The model under review builds one solid part; all positions refer to its coordinate system, in mm. A direction names the side the tool comes from. Coordinates: 2 decimals unless noted, no trailing zeros. Loops run counter-clockwise (first coordinate to the right, second up) from the corner with the lowest first, then second, coordinate; pieces in that order, holes last. Notation, with made-up numbers: (17, -9) - (54, -9) arc R18 cw to (54, 9) - close; hole circle Ø4 at (-24.5, -25). An arc over 180 degrees is marked (long way). Answer in a Markdown table with one row per item. Add a question column.
(1) Mouldability with a two-part tool opening along Y and no side actions: class faces 1 (the flat face through (29.689, 15.675, -12.567)), 2 (the conical face through (-20.821, -93.761, 28.116)), 3 (the flat face through (-8, -77, 28.575)) as +Y half, -Y half, draft (parallel to the pull), parting line (faces both ways), or undercut.
(2) For P1, Ø4, axis at x = -70.5, z = -17.5, coming from the -Y side; P2, Ø6, axis at x = -79, z = 5, coming from the -Y side; P3, Ø15, axis at y = 38, z = -11.5, coming from the +X side, all flat-tipped, find the tip position at first contact; note any pin that passes through.
(3) We need section A-A on z = 18.5. Write out the cut boundary in (x, y) (3 decimals), plus the area to 3 significant figures.
(4) Machinability: for faces 4 (the flat face through (-1.27, 33, -13)), 5 (the cylindrical face through (50.8, -0.4, 12.8)), which of the approach directions +Z, -Z, +X, -X, +Y, -Y give a long, thin tool a straight path to every point of the face, cutting with its end or side? Answer none if there is none.
(5) For line 1 along X through (y, z) = (1, 5.5); line 2 along X through (y, z) = (24, 9); line 3 along X through (y, z) = (-18.5, -4), list the stretches that pass through material, from the lowest coordinate up.
from build123d import *
from OCP.BRepFilletAPI import BRepFilletAPI_MakeChamfer

# Parameters (mm, degrees)
EXTRUDE1_DEPTH          = 28.575
EXTRUDE1_DEPTH_BACK     = 28.575
SKETCH1_R               = 107.95
CHAMFER1_SIZE           = 12.7
CHAMFER1_SIZE2          = 7.332348419
SKETCH2_R               = 60.325
EXTRUDE2_DEPTH          = 6.35
FILLET1_R               = 25.4
SKETCH5_R               = 50.8
EXTRUDE4_DEPTH          = 19.05
SKETCH6_W               = 2.54
SKETCH6_H               = 50.8
EXTRUDE_THIN1_DEPTH     = 19.05
CIRPATTERN2_COUNT       = 6
SKETCH7_R               = 15.875
EXTRUDE5_DEPTH          = 19.05
MIRROR4_COPY_1_SKETCH_W = 2.54
MIRROR4_COPY_1_SKETCH_H = 50.8
MIRROR4_COPY_1_DEPTH    = 19.05
MIRROR4_COPY_2_SKETCH_W = 2.54
MIRROR4_COPY_2_SKETCH_H = 50.8
MIRROR4_COPY_2_DEPTH    = 19.05
MIRROR4_COPY_3_SKETCH_W = 2.54
MIRROR4_COPY_3_SKETCH_H = 50.8
MIRROR4_COPY_3_DEPTH    = 19.05
MIRROR4_COPY_4_SKETCH_W = 2.54
MIRROR4_COPY_4_SKETCH_H = 50.8
MIRROR4_COPY_4_DEPTH    = 19.05
MIRROR4_COPY_5_SKETCH_W = 2.54
MIRROR4_COPY_5_SKETCH_H = 50.8
MIRROR4_COPY_5_DEPTH    = 19.05
FILLET2_R               = 25.4


with BuildPart() as part:
    # Sketch1 → Extrude1 (new, two sides: drawn at the far end of the back side and taken through both)
    with BuildSketch(Plane.XY.offset(-EXTRUDE1_DEPTH_BACK)):
        Circle(SKETCH1_R)
    extrude(amount=EXTRUDE1_DEPTH + EXTRUDE1_DEPTH_BACK)

    # Chamfer1: one chamfer whose edges measure the first distance from different faces: ONE call of the kernel's chamfer builder (chamfer() names one face for all edges)
    chamfer1_edges_1 = [part.edges().sort_by_distance(p)[0] for p in [
        (-107.95, 0, -28.575),
    ]]
    chamfer1_side_1 = [part.faces().sort_by_distance(p)[0] for p in [
        (0, 0, -28.575),
    ]]
    chamfer1_edges_2 = [part.edges().sort_by_distance(p)[0] for p in [
        (-107.95, 0, 28.575),
    ]]
    chamfer1_side_2 = [part.faces().sort_by_distance(p)[0] for p in [
        (0, 0, 28.575),
    ]]
    chamfer1 = BRepFilletAPI_MakeChamfer(part.part.solid().wrapped)
    for e in chamfer1_edges_1:
        chamfer1.Add(CHAMFER1_SIZE, CHAMFER1_SIZE2, e.wrapped, chamfer1_side_1[0].wrapped)  # the first distance lies on this face
    for e in chamfer1_edges_2:
        chamfer1.Add(CHAMFER1_SIZE, CHAMFER1_SIZE2, e.wrapped, chamfer1_side_2[0].wrapped)  # the first distance lies on this face
    add(Compound.cast(chamfer1.Shape()), mode=Mode.REPLACE)

    # Sketch2 → Extrude2 (cut)
    with BuildSketch(Plane.XY.offset(28.575)):
        Circle(SKETCH2_R)
    extrude2 = extrude(amount=-EXTRUDE2_DEPTH, mode=Mode.SUBTRACT)

    # Fillet1
    # the kernel refuses this fillet: 25.4 mm, written as the material it takes off along each edge
    with BuildSketch(Plane(origin=(0, 0, 28.575), x_dir=(1, 0, 0), z_dir=(0, -1, 0))) as fillet1_piece_1:
        with BuildLine():
            CenterArc((77.125520825, -25.4), FILLET1_R, 90, 41.409622109)
            Line((60.325, -6.35), (59.988989583, -5.969))
            ThreePointArc((59.988989583, -5.969), (59.817, -3.175), (59.817, 0))
            Line((59.817, 0), (60.325, 0.508))
            Line((60.325, 0.508), (77.125520825, 0.508))
            Line((77.125520825, 0.508), (77.125520825, 0))
        make_face()
    revolve(axis=Axis((0, 0, 28.575), (0, 0, 1)), mode=Mode.SUBTRACT)

    # Sketch5 → Extrude4 (cut)
    with BuildSketch(Plane.XY.offset(22.225)):
        Circle(SKETCH5_R)
    extrude4 = extrude(amount=-EXTRUDE4_DEPTH, mode=Mode.SUBTRACT)

    # Sketch6 → Extrude-Thin1 (add)
    with BuildSketch(Plane.XY.offset(3.175)):
        with Locations((0, 25.4)):
            Rectangle(SKETCH6_W, SKETCH6_H)
    extrude_thin1 = extrude(amount=EXTRUDE_THIN1_DEPTH)

    # CirPattern2: Extrude-Thin1 ×6 about axis
    cirpattern2_axis = Axis((0, 0, 0), (0, 0, 1))
    for i in range(1, CIRPATTERN2_COUNT):
        add(extrude_thin1.rotate(cirpattern2_axis, i * 360 / CIRPATTERN2_COUNT))

    # Sketch7 → Extrude5 (add)
    with BuildSketch(Plane.XY.offset(22.225)):
        Circle(SKETCH7_R)
    extrude5 = extrude(amount=-EXTRUDE5_DEPTH)

    # Mirror4: Extrude2, Extrude4, Extrude-Thin1, Extrude5 across plane
    add(extrude2.mirror(Plane.XY), mode=Mode.SUBTRACT)
    add(extrude4.mirror(Plane.XY), mode=Mode.SUBTRACT)
    add(extrude_thin1.mirror(Plane.XY))
    add(extrude5.mirror(Plane.XY))

    # Mirror4 copy 1 sketch → Mirror4 copy 1 (add)
    with BuildSketch(Plane(origin=(0, 0, -3.175), x_dir=(0.5000000000000001, 0.8660254037844386, 0), z_dir=(0, 0, -1))):
        with Locations((0, -25.4)):
            Rectangle(MIRROR4_COPY_1_SKETCH_W, MIRROR4_COPY_1_SKETCH_H)
    extrude(amount=MIRROR4_COPY_1_DEPTH)

    # Mirror4 copy 2 sketch → Mirror4 copy 2 (add)
    with BuildSketch(Plane(origin=(0, 0, -3.175), x_dir=(-0.4999999999999998, 0.8660254037844387, 0), z_dir=(0, 0, -1))):
        with Locations((0, -25.4)):
            Rectangle(MIRROR4_COPY_2_SKETCH_W, MIRROR4_COPY_2_SKETCH_H)
    extrude(amount=MIRROR4_COPY_2_DEPTH)

    # Mirror4 copy 3 sketch → Mirror4 copy 3 (add)
    with BuildSketch(Plane(origin=(0, 0, -3.175), x_dir=(-1, 0, 0), z_dir=(0, 0, -1))):
        with Locations((0, -25.4)):
            Rectangle(MIRROR4_COPY_3_SKETCH_W, MIRROR4_COPY_3_SKETCH_H)
    extrude(amount=MIRROR4_COPY_3_DEPTH)

    # Mirror4 copy 4 sketch → Mirror4 copy 4 (add)
    with BuildSketch(Plane(origin=(0, 0, -3.175), x_dir=(-0.5000000000000004, -0.8660254037844384, 0), z_dir=(0, 0, -1))):
        with Locations((0, -25.4)):
            Rectangle(MIRROR4_COPY_4_SKETCH_W, MIRROR4_COPY_4_SKETCH_H)
    extrude(amount=MIRROR4_COPY_4_DEPTH)

    # Mirror4 copy 5 sketch → Mirror4 copy 5 (add)
    with BuildSketch(Plane(origin=(0, 0, -3.175), x_dir=(0.5000000000000001, -0.8660254037844386, 0), z_dir=(0, 0, -1))):
        with Locations((0, -25.4)):
            Rectangle(MIRROR4_COPY_5_SKETCH_W, MIRROR4_COPY_5_SKETCH_H)
    extrude(amount=MIRROR4_COPY_5_DEPTH)

    # Fillet2
    # the kernel refuses this fillet: 25.4 mm, written as the material it takes off along each edge
    with BuildSketch(Plane(origin=(0, 0, -28.575), x_dir=(1, 0, 0), z_dir=(0, -1, 0))) as fillet2_piece_1:
        with BuildLine():
            CenterArc((77.125520825, 25.4), FILLET2_R, 228.590377891, 41.409622109)
            Line((60.325, 6.35), (59.988989583, 5.969))
            ThreePointArc((59.988989583, 5.969), (59.817, 3.175), (59.817, 0))
            Line((59.817, 0), (60.325, -0.508))
            Line((60.325, -0.508), (77.125520825, -0.508))
            Line((77.125520825, -0.508), (77.125520825, 0))
        make_face()
    revolve(axis=Axis((0, 0, -28.575), (0, 0, 1)), mode=Mode.SUBTRACT)


solid = part.part
Outcome:
| question | item | result |
|---|---|---|
| 1 | face 1 | undercut |
| 1 | face 2 | parting line |
| 1 | face 3 | draft |
| 2 | P1 | y = -83.43 |
| 2 | P2 | y = -76.66 |
| 2 | P3 | x = 103.55 |
| 3 | outline | circle Ø215.9 at (0, 0); hole (-44.615, -24.292) - (-14.339, -6.812) arc R15.875 cw to (-14.339, 6.812) - (-44.615, 24.292) arc R50.8 ccw to start; hole (-43.345, -26.492) arc R50.8 ccw to (-1.27, -50.784) - (-1.27, -15.824) arc R15.875 cw to (-13.069, -9.012) - close; hole (-43.345, 26.492) - (-13.069, 9.012) arc R15.875 cw to (-1.27, 15.824) - (-1.27, 50.784) arc R50.8 ccw to start; hole (1.27, -50.784) arc R50.8 ccw to (43.345, -26.492) - (13.069, -9.012) arc R15.875 cw to (1.27, -15.824) - close; hole (1.27, 15.824) arc R15.875 cw to (13.069, 9.012) - (43.345, 26.492) arc R50.8 ccw to (1.27, 50.784) - close; hole (14.339, -6.812) - (44.615, -24.292) arc R50.8 ccw to (44.615, 24.292) - (14.339, 6.812) arc R15.875 cw to start |
| 3 | area | 29,800 mm² |
| 4 | face 4 | -Z |
| 4 | face 5 | +Z |
| 5 | line 1 | -107.95 to -50.79, -15.84 to 15.84, 50.79 to 107.95 |
| 5 | line 2 | -105.25 to -44.77, -44.11 to -39.03, -1.27 to 1.27, 39.03 to 44.11, 44.77 to 105.25 |
| 5 | line 3 | -106.35 to -47.31, -34.58 to -29.5, -1.27 to 1.27, 29.5 to 34.58, 47.31 to 106.35 |
